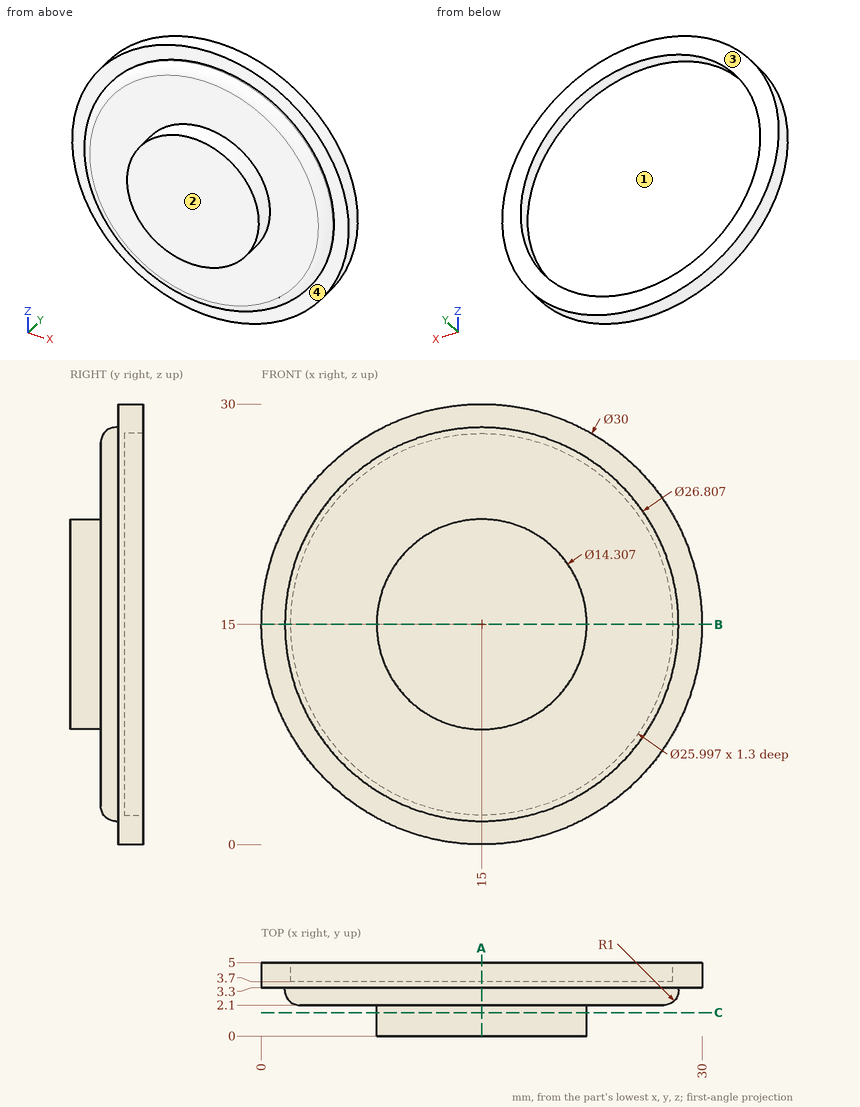
Geometry: see drawing. Coordinates: mm, zero at the bounding-box minimum. A direction names the side the tool comes from. Coordinates: 2 decimals unless noted, no trailing zeros. Loops run counter-clockwise (first coordinate to the right, second up) from the corner with the lowest first, then second, coordinate; pieces in that order, holes last.
(1) Section C-C on y = 1.6. Return the cut outline in (x, z).
(2) Material intervals for probe 1 along X at (y, z) = (4.45, 15); probe 2 along Y at (x, z) = (14, 7.5); probe 3 along Y at (x, z) = (11.75, 8.75), sorted ascending.
(3) Section A-A on x = 15. Return the cut outline in (y, z).
(4) First-contact query: pin 1 Ø8 at (x, z) = (18.5, 14.5) entering from +Y; pin 2 Ø1.5 at (y, z) = (3.5, 21.5) entering from +X (1 decimal); pin 3 Ø4 at (x, z) = (26, 6) entering from -Y. Flat tips, straight axial feed; report the tip coordinate or a pass-through.
(5) Set-up query: the marked faces 3 and 4. Return all of +Z, -Z, +X, -X, +Y, -Y with unobstructed straight access to the full face (end or side cutting, diameter ignored); none if empty.
(6) Section B-B on z = 15. Return the cut outline in (x, y).
(7) Pull-direction query (X, two-part tool) for the marked faces 1 and 2; classes: released by +X, released by -X, zero draft, split by the parting line, or undercut.
Data:
1. outline: circle Ø14.31 at (15, 15)
2. probe 1: x = 0 to 2, 28 to 30
2. probe 2: y = 2.1 to 3.7
2. probe 3: y = 0 to 3.7
3. outline: (0, 7.85) - (2.1, 7.85) - (2.1, 2.6) arc R1 ccw to (3.1, 1.6) - (3.3, 1.6) - (3.3, 0) - (5, 0) - (5, 2) - (3.7, 2) - (3.7, 28) - (5, 28) - (5, 30) - (3.3, 30) - (3.3, 28.4) - (3.1, 28.4) arc R1 ccw to (2.1, 27.4) - (2.1, 22.15) - (0, 22.15) - close
4. pin 1: stops at y = 3.7
4. pin 2: stops at x = 28.9
4. pin 3: stops at y = 2.1
5. face 3: +Z, -Z, +X, -X, +Y
5. face 4: -Y
6. outline: (0, 3.3) - (1.6, 3.3) - (1.6, 3.1) arc R1 ccw to (2.6, 2.1) - (7.85, 2.1) - (7.85, 0) - (22.15, 0) - (22.15, 2.1) - (27.4, 2.1) arc R1 ccw to (28.4, 3.1) - (28.4, 3.3) - (30, 3.3) - (30, 5) - (28, 5) - (28, 3.7) - (2, 3.7) - (2, 5) - (0, 5) - close
7. face 1: undercut
7. face 2: zero draft
